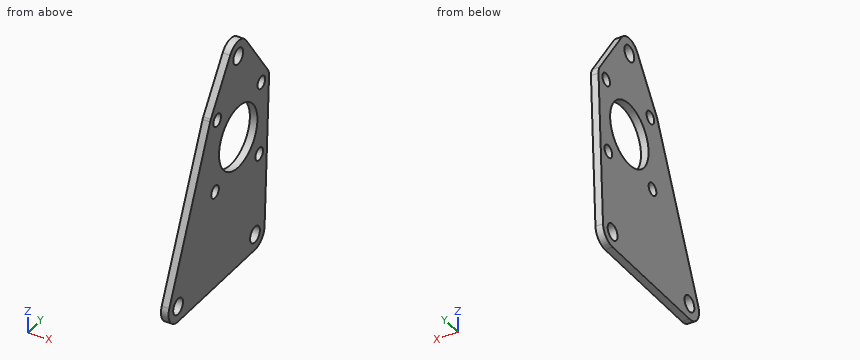
```python
from build123d import *

# Parameters (mm, degrees)
SKETCH1_R             = 2.4384
SKETCH1_R_2           = 9.525
BASE_FLANGE1_DEPTH    = 2.286
F_6_CLEARANCE_HOLE1_D = 3.7973


# Sheet-metal steps are written as plain solids
with BuildPart() as part:
    # Sketch1 → Base-Flange1 (new body)
    with BuildSketch(Plane(origin=(0, 0, 0), x_dir=(0, 0, -1), z_dir=(1, 0, 0))):
        with BuildLine():
            Line((4.7625, 38.1), (4.7625, 0))
            ThreePointArc((4.7625, 0), (2.61262586, -3.981908131), (-1.896016479, -4.368813084))
            Line((-1.896016479, -4.368813084), (-48.551698058, 15.879235852))
            ThreePointArc((-48.551698058, 15.879235852), (-48.856590074, 16.028021212), (-49.147038032, 16.203338662))
            Line((-49.147038032, 16.203338662), (-63.600191446, 25.830515429))
            ThreePointArc((-63.600191446, 25.830515429), (-65.722355809, 29.757140553), (-63.661556753, 33.716316439))
            Line((-63.661556753, 33.716316439), (-48.141159083, 44.406778026))
            ThreePointArc((-48.141159083, 44.406778026), (-47.023714737, 44.933314584), (-45.796546729, 45.074669792))
            Line((-45.796546729, 45.074669792), (0.229208689, 42.856981146))
            ThreePointArc((0.229208689, 42.856981146), (3.447681296, 41.385559303), (4.7625, 38.1))
        make_face()
        with Locations((0, 38.1)):
            Circle(SKETCH1_R, mode=Mode.SUBTRACT)
        Circle(SKETCH1_R, mode=Mode.SUBTRACT)
        with Locations((-60.96, 29.7942)):
            Circle(SKETCH1_R, mode=Mode.SUBTRACT)
        with Locations((-35.56, 29.7942)):
            Circle(SKETCH1_R_2, mode=Mode.SUBTRACT)
    extrude(amount=-BASE_FLANGE1_DEPTH)

    # #6 Clearance Hole1 (through all)
    with Locations(Plane(origin=(0, 0, 0), x_dir=(0, 0, -1), z_dir=(1, 0, 0))):
        with Locations((-24.085115125, 40.214113681), (-45.979913681, 41.269084875), (-25.140086319, 18.319315125), (-47.034884875, 19.374286319)):
            Hole(F_6_CLEARANCE_HOLE1_D / 2)


solid = part.part
```
CAD build for the part. Positions are in the model's coordinates, mm. Coordinates: 2 decimals unless noted, no trailing zeros. Order: outer loops, then holes, each group sorted by start corner. A loop starts at its lowest first (then second) coordinate and runs counter-clockwise, first axis right, second up. Notation, with made-up numbers: (40, 1) -> (64, 1) arc R28 cw to (64, 38) -> close; hole circle Ø4 at (22.5, 2.5). An arc over 180 degrees is marked (long way). Use one line per item in the form item = value. Start each with the question number.
1) Band-saw the part on B-B on x = -1.4. State how many separate pieces and enclosed holes the cut face has, then the cut area to 3 significant figures.
2) Drill centre lines: L1, parallel to Y at x = -0.85, z = 0; L2, parallel to Z at x = -0.35, y = 29.5; L3, parallel to Y at x = -1.6, z = 1.5. Where is each one in solid material? Low to high. Write a range as [from, to].
3) Band-saw the part on C-C on y = 23.5. Give the cut face in (x, z), then the cut area to 3 significant figures.
4) Band-saw the part on D-D on z = 35.56. Give the cut face in (x, y).
5) Band-saw the part on A-A on y = 28.5. Give the cut face in (x, z).
Entries:
q1.separate_pieces = 1
q1.enclosed_holes = 8
q1.area = 1,990 mm2
q2.L1 = [-4.76, -2.44], [2.44, 35.66], [40.54, 42.87]
q2.L2 = [-4.76, 26.04], [45.08, 58.54], [63.38, 65.71]
q2.L3 = [-4.52, -1.92], [1.92, 36.18], [40.02, 42.94]
q3.outline = (-2.29, -4.76) -> (0, -4.76) -> (0, 28.41) -> (-2.29, 28.41) -> close; (-2.29, 42.71) -> (0, 42.71) -> (0, 60.1) -> (-2.29, 60.1) -> close
q3.area = 116 mm2
q4.outline = (-2.29, 10.24) -> (0, 10.24) -> (0, 20.27) -> (-2.29, 20.27) -> close; (-2.29, 39.32) -> (0, 39.32) -> (0, 44.58) -> (-2.29, 44.58) -> close
q5.outline = (-2.29, -4.76) -> (0, -4.76) -> (0, 26.12) -> (-2.29, 26.12) -> close; (-2.29, 45) -> (0, 45) -> (0, 58.89) -> (-2.29, 58.89) -> close; (-2.29, 63.03) -> (0, 63.03) -> (0, 65.54) -> (-2.29, 65.54) -> close
